Geometry check sheet. Reference: the model listing, model coordinates, mm. A direction names the side the tool comes from. Coordinates: 2 decimals unless noted, no trailing zeros. Loops run counter-clockwise (first coordinate to the right, second up) from the corner with the lowest first, then second, coordinate; pieces in that order, holes last.
from build123d import *

# Parameters (mm, degrees)
BOSS_EXTRUDE4_DEPTH = 304.8
SHELL1_T            = -2.54
SKETCH3_W           = 50.8
SKETCH3_H           = 50.8
BOSS_EXTRUDE5_DEPTH = 381
SKETCH4_W           = 63.5
SKETCH4_H           = 63.5
BOSS_EXTRUDE6_DEPTH = 2.54
SKETCH5_W           = 5.08
SKETCH5_H           = 63.5
SKETCH5_H_2         = 63.212567158
BOSS_EXTRUDE7_DEPTH = 50.8
BOSS_EXTRUDE8_REACH = 1036.844
SKETCH6_R           = 19.05
SKETCH7_W           = 30.48
SKETCH7_H           = 279.4
CUT_EXTRUDE1_DEPTH  = 431.8


with BuildPart() as part:
    # Sketch2 → Boss-Extrude4 (new body)
    with BuildSketch(Plane.XY):
        Polygon((489.227839492, 0), (104.27186579, 0), (104.27186579, 914.4), (489.227839492, 914.4), (489.227839492, 809.506234414), (196.520335525, 809.506234414), (196.520335525, 526.127227386), (477.826343233, 526.127227386), (477.826343233, 421.2334618), (196.520335525, 421.2334618), (196.520335525, 106.34486511), (489.227839492, 106.34486511), align=None)
    extrude(amount=-BOSS_EXTRUDE4_DEPTH)

    # Shell1
    shell1_openings = [part.faces().sort_by_distance(p)[0] for p in [
        (249.504622919, 459.117899523, -304.8),
    ]]
    offset(amount=SHELL1_T, openings=shell1_openings, kind=Kind.INTERSECTION)

    # Sketch3 → Boss-Extrude5 (add)
    with BuildSketch(Plane(origin=(0, 0, -2.54), x_dir=(-1, 0, 0), z_dir=(0, 0, -1))):
        with Locations((-294.77186579, 473.328769938)):
            Rectangle(SKETCH3_W, SKETCH3_H)
    extrude(amount=BOSS_EXTRUDE5_DEPTH)

    # Sketch4 → Boss-Extrude6 (add)
    with BuildSketch(Plane(origin=(0, 0, -383.54), x_dir=(-1, 0, 0), z_dir=(0, 0, -1))):
        with Locations((-294.77186579, 473.328769938)):
            Rectangle(SKETCH4_W, SKETCH4_H)
    extrude(amount=BOSS_EXTRUDE6_DEPTH)

    # Sketch5 → Boss-Extrude7 (add)
    with BuildSketch(Plane(origin=(0, 0, -386.08), x_dir=(-1, 0, 0), z_dir=(0, 0, -1))):
        with Locations((-316.36186579, 473.328769938)):
            Rectangle(SKETCH5_W, SKETCH5_H)
        with Locations((-273.18186579, 473.472486359)):
            Rectangle(SKETCH5_W, SKETCH5_H_2)
    extrude(amount=BOSS_EXTRUDE7_DEPTH)

    # Sketch6 → Boss-Extrude8 (add, up to next)
    with BuildSketch(Plane.ZY.offset(-313.82186579), mode=Mode.PRIVATE) as boss_extrude8_sk1:
        with Locations(Location((-411.48, 473.328769938, 0), (0, 0, 180))):
            Circle(SKETCH6_R)
    boss_extrude8_tool1 = extrude(boss_extrude8_sk1.sketch, amount=BOSS_EXTRUDE8_REACH, mode=Mode.PRIVATE) - part.part
    add(boss_extrude8_tool1.solids().sort_by_distance((313.821866, 473.32877, -411.48))[0])

    # Sketch7 → Cut-Extrude1 (cut)
    with BuildSketch(Plane.XZ):
        with Locations((297.31186579, -165.1)):
            Rectangle(SKETCH7_W, SKETCH7_H)
    extrude(amount=-CUT_EXTRUDE1_DEPTH, mode=Mode.SUBTRACT)


solid = part.part
1) Section check C-C on y = 395. Record the cut outline in (x, z).
Data:
outline: (104.27, -304.8) - (106.81, -304.8) - (106.81, -2.54) - (193.98, -2.54) - (193.98, -304.8) - (196.52, -304.8) - (196.52, 0) - (104.27, 0) - close
2) Depth check by flat-ended pin: pin 1 (10 mm diameter, centred on x = 170, y = 448.5, fed in from -Z); pin 2 (1 mm diameter, centred on y = 334.5, z = -243.5, fed in from +X); pin 3 (0.8 mm diameter, centred on y = 459, z = -384.5, fed in from +X). Enter the tip coordinate at first touch or a pass-through.
Data:
pin 1: stops at z = -2.54
pin 2: stops at x = 196.52
pin 3: stops at x = 326.52
3) Mould release check, pull along X, two halves, no side actions. Record for faces 4 (the flat face through (342, 2.54, -152)), 5 (the flat face through (104.272, 451, -150)), 6 (the flat face through (345, 809.506, -150)): +X half, -X half, draft (parallel to the pull), parting line (faces both ways), or undercut.
Data:
face 4: undercut
face 5: -X half
face 6: draft
4) Access from +Z, -Z, +X, -X, +Y, -Y to the whole of each face (thin tool, end or side, straight path). Record for faces 1 (the flat face through (318.902, 473, -411)), 2 (the cylindrical face through (295.039, 491.926, -407.35)), 3 (the flat face through (316, 441.579, -402)).
Data:
face 1: -Z, +X, +Y, -Y
face 2: none
face 3: -Z, +X, -X, -Y
5) Section check D-D on z = -256.5. Count the separate pieces of the cut face and the enclosed holes in it, and give its area (3 significant figures).
Data:
separate pieces: 4
enclosed holes: 0
area: 11,800 mm2
6) Section check A-A on x = 463. Record the cut outline in (y, z).
Data:
outline: (0, -304.8) - (2.54, -304.8) - (2.54, -2.54) - (103.8, -2.54) - (103.8, -304.8) - (106.34, -304.8) - (106.34, 0) - (0, 0) - close; (421.23, -304.8) - (423.77, -304.8) - (423.77, -2.54) - (523.59, -2.54) - (523.59, -304.8) - (526.13, -304.8) - (526.13, 0) - (421.23, 0) - close; (809.51, -304.8) - (812.05, -304.8) - (812.05, -2.54) - (911.86, -2.54) - (911.86, -304.8) - (914.4, -304.8) - (914.4, 0) - (809.51, 0) - close
7) Material ranges on probe 1 along Y at (x, z) = (231, -66); probe 2 along X at (y, z) = (104, -53); probe 3 along Y at (x, z) = (193.5, -86.5), recorded low to high.
Data:
probe 1: y = 0 to 2.54, 103.8 to 106.34, 421.23 to 423.77, 523.59 to 526.13, 809.51 to 812.05, 911.86 to 914.4
probe 2: x = 104.27 to 106.81, 193.98 to 282.07, 312.55 to 489.23
probe 3: y = 0 to 2.54, 911.86 to 914.4
8) Section check B-B on z = -411.48. Record the cut outline in (x, y), and give its area (3 significant figures).
Data:
outline: (270.64, 441.87) - (275.72, 441.87) - (275.72, 454.28) - (313.82, 454.28) - (313.82, 441.58) - (318.9, 441.58) - (318.9, 505.08) - (313.82, 505.08) - (313.82, 492.38) - (275.72, 492.38) - (275.72, 505.08) - (270.64, 505.08) - close
area: 2,100 mm2
